Geometry check sheet. Reference: the model listing, model coordinates, mm. A direction names the side the tool comes from. Coordinates: 2 decimals unless noted, no trailing zeros. Loops run counter-clockwise (first coordinate to the right, second up) from the corner with the lowest first, then second, coordinate; pieces in that order, holes last.
from build123d import *

# Parameters (mm, degrees)
MODEL_R                 = 5
SALIENTE_EXTRUIR1_DEPTH = 3


with BuildPart() as part:
    # Model → Saliente-Extruir1 (new body)
    with BuildSketch(Plane.XY):
        Polygon((124.511184003, 58.317312114), (112.50181664, 58.326235146), (112.501811813, 36.503581249), (112.501804141, 1.819115993), (112.501801747, -9.003305006), (112.501792152, -52.377623741), (137.401805699, -52.391743595), (137.401805699, -55.885276943), (145.601805699, -55.885276943), (145.601805699, -52.385276943), (162.401805699, -52.385276943), (162.401805699, -55.885276943), (170.601805699, -55.885276943), (170.601805699, -52.385276943), (195.501819246, -52.392930144), (195.275424073, 79.124358077), (158.510749751, 79.124374738), (158.510749751, 67.325142582), (135.310749751, 67.32643696), (135.310749751, 79.124374745), (124.511184003, 79.124374745), align=None)
        Polygon((144.00179591, -43.389548344), (144.00179591, -49.389548344), (133.00179591, -49.389548344), (133.00179591, -43.389548344), (128.50179591, -43.389548344), (128.50179591, -35.389548344), (133.00179591, -35.389548344), (133.00179591, -29.389548344), (144.00179591, -29.389548344), (144.00179591, -35.389548344), (148.50179591, -35.389548344), (148.50179591, -43.389548344), align=None, mode=Mode.SUBTRACT)
        with Locations((154.001805699, -29.885276943)):
            Circle(MODEL_R, mode=Mode.SUBTRACT)
        Polygon((175.001819246, -43.389558962), (175.001819246, -49.389558962), (164.001819246, -49.389558962), (164.001819246, -43.389558962), (159.501819246, -43.389558962), (159.501819246, -35.389558962), (164.001819246, -35.389558962), (164.001819246, -29.389558962), (175.001819246, -29.389558962), (175.001819246, -35.389558962), (179.501819246, -35.389558962), (179.501819246, -43.389558962), align=None, mode=Mode.SUBTRACT)
    extrude(amount=SALIENTE_EXTRUIR1_DEPTH)


solid = part.part
1) Section check A-A on x = 165.5. Record the cut outline in (y, z).
Data:
outline: (-55.89, 0) - (-49.39, 0) - (-49.39, 3) - (-55.89, 3) - close; (-29.39, 0) - (79.12, 0) - (79.12, 3) - (-29.39, 3) - close
2) Depth check by flat-ended pin: pin 1 (1 mm diameter, centred on y = 46.5, z = 1.5, fed in from +X); pin 2 (1.5 mm diameter, centred on x = 177, z = 1, fed in from -Y); pin 3 (0.9 mm diameter, centred on y = -33.5, z = 1.5, fed in from +X). Enter the tip coordinate at first touch or a pass-through.
Data:
pin 1: stops at x = 195.33
pin 2: stops at y = -52.39
pin 3: stops at x = 195.47
3) Section check B-B on y = -33. Record the cut outline in (x, z), and give its area (3 significant figures).
Data:
outline: (112.5, 0) - (133, 0) - (133, 3) - (112.5, 3) - close; (144, 0) - (150.09, 0) - (150.09, 3) - (144, 3) - close; (157.91, 0) - (164, 0) - (164, 3) - (157.91, 3) - close; (175, 0) - (195.47, 0) - (195.47, 3) - (175, 3) - close
area: 159 mm2
4) Material ranges on probe 1 along Y at (x, z) = (143, 2.5); probe 2 along Y at (x, z) = (146, 0.8); probe 3 along X at (y, z) = (67.5, 2.1), recorded low to high.
Data:
probe 1: y = -55.89 to -49.39, -29.39 to 67.33
probe 2: y = -52.39 to -43.39, -35.39 to 67.33
probe 3: x = 124.51 to 135.31, 158.51 to 195.3
5) Section check C-C on y = 69.5. Record the cut outline in (x, z), and give its area (3 significant figures).
Data:
outline: (124.51, 0) - (135.31, 0) - (135.31, 3) - (124.51, 3) - close; (158.51, 0) - (195.29, 0) - (195.29, 3) - (158.51, 3) - close
area: 143 mm2
6) Mould release check, pull along X, two halves, no side actions. Record for faces 5 (the flat face through (146, -43.39, 1)), 6 (the flat face through (130, 79.124, 1)), 7 (the flat face through (137.402, -54, 1)): +X half, -X half, draft (parallel to the pull), parting line (faces both ways), or undercut.
Data:
face 5: undercut
face 6: draft
face 7: -X half
7) Access from +Z, -Z, +X, -X, +Y, -Y to the whole of each face (thin tool, end or side, straight path). Record for faces 1 (the flat face through (164.002, -32, 1)), 2 (the flat face through (145.602, -54, 1)), 3 (the flat face through (124.511, 69, 1)), 4 (the flat face through (170.602, -54, 1)).
Data:
face 1: +Z, -Z
face 2: +Z, -Z, -Y
face 3: +Z, -Z, -X, +Y
face 4: +Z, -Z, +X, -Y
8) Section check D-D on z = 1.3. Count the separate pieces of the cut face and the enclosed holes in it, and give its area (3 significant figures).
Data:
separate pieces: 1
enclosed holes: 3
area: 9,770 mm2
